Work out the finished part from the listing and answer in its coordinate system (mm). Face numbers are marked on the shaded views. A direction names the side the tool comes from. Give positions to 0.01 mm unless a question says otherwise; leave off trailing zeros. Write each loop counter-clockwise with the first axis right and the second up, starting at its lowest first coordinate (ties: lowest second). Pieces come first, ordered by that corner, then holes.
1) Given pin 1 Ø2.5 at (x, y) = (7.5, -37.5) entering from +Z; pin 2 Ø1.5 at (x, z) = (3.5, 21.5) entering from -Y; pin 3 Ø8 at (y, z) = (9.5, 29) entering from +X, each flat-ended and moving along its own axis, determine where each tip first touches the part or whether it passes through.
2) Find section B-B (x = -7.5). Determine the outline of the cut face in (y, z), plus the area to 3 significant figures.
3) Find section D-D (z = 9). Determine the outline of the cut face in (x, y).
4) Find section C-C (y = -37.5). Determine the outline of the cut face in (x, z), plus the area to 3 significant figures.
5) A tool of negligible diameter and unlimited length cuts with its end or side. For the marked faces 1 and 2, from which of +Z, -Z, +X, -X, +Y, -Y can it reach the whole face along a straight path? Write none if from no direction.
6) Straight lines are drawn through the part: probe 1 along Y at (x, z) = (-7.5, 47); probe 2 along X at (y, z) = (37, 48); probe 3 along Z at (x, y) = (8, 22). For each, find the intervals that lie inside material, in ascending order.
7) Find section A-A (y = 0). Determine the outline of the cut face in (x, z), plus the area to 3 significant figures.
Autodesk Inventor part; units mm, degrees
ref_plane "Plano de trabajo2" through (7.156, -49.9529, 91.9135) normal (-0.1189, 0.9929, 0) x (-0.9929, -0.1189, 0)
ref_plane "YZ Plane" through (0, 0, 0) normal (1, 0, 0) x (0, 1, 0)
ref_plane "XZ Plane" through (0, 0, 0) normal (0, 1, 0) x (-1, 0, 0)
ref_plane "Plano de trabajo2" through (7.156, -49.9529, 91.9135) normal (-0.1189, 0.9929, 0) x (-0.9929, -0.1189, 0)
ref_plane "Plano de trabajo5" through (0, 0, 40) normal (0, 0, 1) x (1, 0, 0)
sketch "Boceto7" plane through (0, 0, 40) normal (0, 0, 1) x (1, 0, 0)
  line L0 (-7.5, 37.5) -> (7.5, 37.5)
  line L1 (7.5, 37.5) -> (7.5, -37.5)
  line L2 (7.5, -37.5) -> (-7.5, -37.5)
  line L3 (-7.5, -37.5) -> (-7.5, 37.5)
  line L4 (-7.5, 37.5) -> (7.5, -37.5) construction
  line L5 (7.5, 37.5) -> (-7.5, -37.5) construction
  line L6 (-11.5, 41.5) -> (11.5, 41.5)
  line L7 (11.5, 41.5) -> (11.5, -41.5)
  line L8 (11.5, -41.5) -> (-11.5, -41.5)
  line L9 (-11.5, -41.5) -> (-11.5, 41.5)
  line L10 (-11.5, 41.5) -> (11.5, -41.5) construction
  line L11 (11.5, 41.5) -> (-11.5, -41.5) construction
  point P0 (0, 0)
  dimension "d18" = 15
  dimension "d19" = 75
  dimension "d32" = 23
  dimension "d33" = 83
extrude "Extrusión5" add sketch "Boceto7" along normal blind 10 contours L0 L1 L2 L3 | L6 L7 L8 L9
ref_plane "Plano de trabajo4" through (0, 0, 40) normal (0, 0, 1) x (1, 0, 0)
sketch "Boceto10" plane through (0, 0, 50) normal (0, 0, 1) x (1, 0, 0)
  line L0 (7.5, -37.5) -> (7.5, 37.5)
  line L1 (7.5, 37.5) -> (0, 37.5)
  line L2 (7.5, 37.5) -> (-7.5, 37.5)
  line L3 (3.75, 37.5) -> (3.75, 37.5)
  line L4 (0, 37.5) -> (0, 32.43)
  line L5 (0, 0) -> (7.5, 0)
  line L6 (0, 37.5) -> (7.5, 37.5)
  circle A0 centre (7.5, 37.5) radius 2.022
  circle A1 centre (-7.5, 37.5) radius 2.022
  circle A2 centre (7.5, -37.5) radius 2.022
  circle A3 centre (-7.5, -37.5) radius 2.022
  dimension "d28" = 0
  dimension "d35" = 7.5
  dimension "d36" = 4.044
  dimension "d37" = 4.044
extrude "Extrusión6" cut sketch "Boceto10" against normal blind 8
sketch "Boceto11" plane through (0, 0, 40) normal (0, 0, -1) x (-1, 0, 0)
  circle A0 centre (0, 0) radius 10
  dimension "d38" = 20
extrude "Extrusión7" add sketch "Boceto11" along normal blind 40
properties part number "UNION_B"
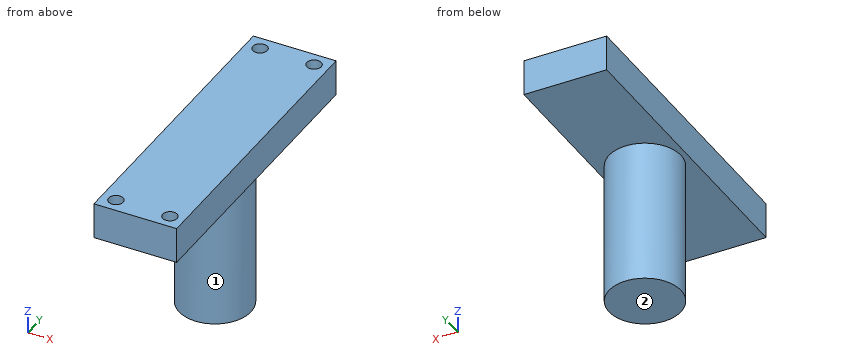
Results:
1. pin 1: stops at z = 42
1. pin 2: stops at y = -9.61
1. pin 3: stops at x = 8.35
2. outline: (-41.5, 40) - (-6.61, 40) - (-6.61, 0) - (6.61, 0) - (6.61, 40) - (41.5, 40) - (41.5, 50) - (39.52, 50) - (39.52, 42) - (35.48, 42) - (35.48, 50) - (-35.48, 50) - (-35.48, 42) - (-39.52, 42) - (-39.52, 50) - (-41.5, 50) - close
2. area: 1,290 mm2
3. outline: circle Ø20 at (0, 0)
4. outline: (-11.5, 40) - (11.5, 40) - (11.5, 50) - (9.52, 50) - (9.52, 42) - (5.48, 42) - (5.48, 50) - (-5.48, 50) - (-5.48, 42) - (-9.52, 42) - (-9.52, 50) - (-11.5, 50) - close
4. area: 165 mm2
5. face 1: -Z
5. face 2: -Z, +X, -X, +Y, -Y
6. probe 1: y = -41.5 to -39.52, -35.48 to 35.48, 39.52 to 41.5
6. probe 2: x = -11.5 to -9.46, -5.54 to 5.54, 9.46 to 11.5
6. probe 3: z = 40 to 50
7. outline: (-11.5, 40) - (-10, 40) - (-10, 0) - (10, 0) - (10, 40) - (11.5, 40) - (11.5, 50) - (-11.5, 50) - close
7. area: 1,030 mm2
